For this review, take the finished solid that the model builds, in its own axes (mm). Face numbers are marked on the shaded views. A direction names the side the tool comes from. Round coordinates to 2 decimals unless told otherwise and drop trailing zeros. Write each loop counter-clockwise with the first axis right and the second up, starting at its lowest first coordinate (ties: lowest second). Pieces come first, ordered by that corner, then holes. Notation, with made-up numbers: (4, -7.75) -> (44, -7.75) arc R22 cw to (44, 21.25) -> close; hole circle Ø4 at (26.25, -29.5). An arc over 180 degrees is marked (long way). Answer in a Markdown table with one row per item. Add a question column.
Autodesk Inventor part; units mm, degrees
ref_plane "YZ Plane" through (0, 0, 0) normal (1, 0, 0) x (0, 1, 0)
ref_plane "XZ Plane" through (0, 0, 0) normal (0, 1, 0) x (-1, 0, 0)
ref_plane "XY Plane" through (0, 0, 0) normal (0, 0, 1) x (1, 0, 0)
sketch "スケッチ1" plane through (0, 0, 0) normal (1, 0, 0) x (0, 1, 0)
  line L0 (-12.5, 12.5) -> (12.5, 12.5)
  line L1 (12.5, 12.5) -> (12.5, -12.5)
  line L2 (12.5, -12.5) -> (-12.5, -12.5)
  line L3 (-12.5, -12.5) -> (-12.5, 12.5)
  line L4 (-12.5, 12.5) -> (12.5, -12.5) construction
  line L5 (12.5, 12.5) -> (-12.5, -12.5) construction
  line L6 (-10.2, 10.2) -> (10.2, 10.2)
  line L7 (10.2, 10.2) -> (10.2, -10.2)
  line L8 (10.2, -10.2) -> (-10.2, -10.2)
  line L9 (-10.2, -10.2) -> (-10.2, 10.2)
  line L10 (-10.2, 10.2) -> (10.2, -10.2) construction
  line L11 (10.2, 10.2) -> (-10.2, -10.2) construction
  point P0 (0, 0)
  dimension "d0" = 25
  dimension "d1" = 25
  dimension "d2" = 2.3
extrude "押し出し1" add sketch "スケッチ1" along normal blind 30
sketch "スケッチ2" plane through (0, -12.5, 12.5) normal (0, 0, 1) x (1, 0, 0)
  circle A0 centre (10, 12.5) radius 2.5
  line L0 (0, 0) -> (0, 25)
  line L1 (0, 0) -> (30, 0)
  point P0 (0, 12.5)
  dimension "d5" = 5
  dimension "d6" = 10
  dimension "d7" = 12.5
extrude "押し出し2" cut sketch "スケッチ2" against normal through all
properties part number "bracket1(body)" material "鉄、可鍛鉄"
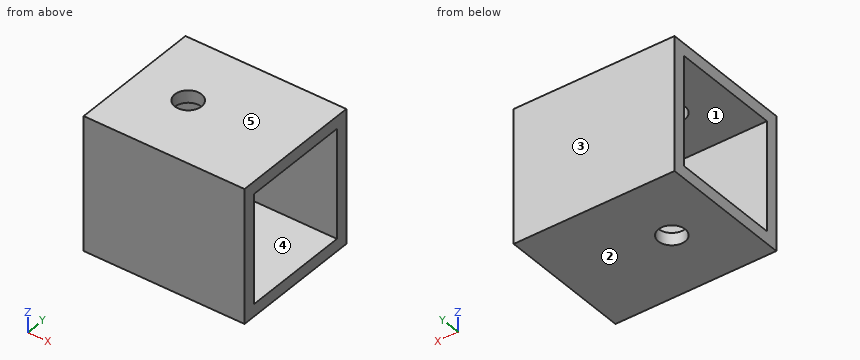
1. Tool access review of the marked faces 1 and 2: name each direction out of +Z, -Z, +X, -X, +Y, -Y from which nothing blocks a thin tool from reaching the whole face with its end or side.
2. For L1, parallel to Z at x = 22, y = 6.5; L2, parallel to Y at x = 10, z = 11.3, list the stretches that pass through material, from the lowest coordinate up. Write a range as [from, to].
3. Clearance check with a flat-ended pin moving along its axis: pin 1 Ø6.5 at (x, y) = (10, 0) entering from +Z. State where the tip first meets the part, or that it passes through.
4. We need section B-B (y = 0). Write out the cut boundary in (x, z).
5. The part is to be moulded in two halves that separate along Y. For the marked faces 3, 4 and 5, say which applies: pulls with the +Y half, pulls with the -Y half, needs draft (parallel to the pull), parting line crosses it, or undercut.
6. We need section A-A (x = 10). Write out the cut boundary in (y, z), plus the area to 3 significant figures.
7. We need section C-C (z = 8.5). Write out the cut boundary in (x, y), plus the area to 3 significant figures.
Response:
| question | item | result |
|---|---|---|
| 1 | face 1 | +X, -X |
| 1 | face 2 | -Z, +X, -X, +Y, -Y |
| 2 | L1 | [-12.5, -10.2], [10.2, 12.5] |
| 2 | L2 | [-12.5, -2.5], [2.5, 12.5] |
| 3 | pin 1 | z = 12.5 |
| 4 | outline | (0, -12.5) -> (7.5, -12.5) -> (7.5, -10.2) -> (0, -10.2) -> close; (0, 10.2) -> (7.5, 10.2) -> (7.5, 12.5) -> (0, 12.5) -> close; (12.5, -12.5) -> (30, -12.5) -> (30, -10.2) -> (12.5, -10.2) -> close; (12.5, 10.2) -> (30, 10.2) -> (30, 12.5) -> (12.5, 12.5) -> close |
| 5 | face 3 | pulls with the +Y half |
| 5 | face 4 | undercut |
| 5 | face 5 | needs draft |
| 6 | outline | (-12.5, -12.5) -> (-2.5, -12.5) -> (-2.5, -10.2) -> (-10.2, -10.2) -> (-10.2, 10.2) -> (-2.5, 10.2) -> (-2.5, 12.5) -> (-12.5, 12.5) -> close; (2.5, -12.5) -> (12.5, -12.5) -> (12.5, 12.5) -> (2.5, 12.5) -> (2.5, 10.2) -> (10.2, 10.2) -> (10.2, -10.2) -> (2.5, -10.2) -> close |
| 6 | area | 186 mm2 |
| 7 | outline | (0, -12.5) -> (30, -12.5) -> (30, -10.2) -> (0, -10.2) -> close; (0, 10.2) -> (30, 10.2) -> (30, 12.5) -> (0, 12.5) -> close |
| 7 | area | 138 mm2 |
